```python
from build123d import *

# Parameters (mm, degrees)
SKETCH_1_W           = 36
SKETCH_1_H           = 219
EXTRUDE_1_DEPTH      = 37
SKETCH_2_W           = 80.767995678
SKETCH_2_H           = 159
CUT_EXTRUDE_1_DEPTH  = 117.975424769
CUT_EXTRUDE_START    = 10
SKETCH_9_W           = 26
SKETCH_9_H           = 219
CUT_EXTRUDE_7_DEPTH  = 17
SKETCH_10_W          = 12
SKETCH_10_H          = 236
CUT_EXTRUDE_8_DEPTH  = 17
CUT_EXTRUDE_START_2  = 37
SKETCH_11_R          = 3.5
CUT_EXTRUDE_11_DEPTH = 17
SKETCH_25_R          = 15
EXTRUDE_3_DEPTH      = 60
CUT_EXTRUDE_START_3  = -78
SKETCH_26_R          = 11
CUT_EXTRUDE_13_DEPTH = 3


with BuildPart() as part:
    # 스케치1 → 보스-돌출1 (new body)
    with BuildSketch(Plane.XY):
        Rectangle(SKETCH_1_W, SKETCH_1_H)
    extrude(amount=EXTRUDE_1_DEPTH)

    # 스케치2 → 컷-돌출1 (cut, through all)
    with BuildSketch(Plane.XY):
        with Locations((32.383997839, -3)):
            Rectangle(SKETCH_2_W, SKETCH_2_H)
    extrude(amount=CUT_EXTRUDE_1_DEPTH, mode=Mode.SUBTRACT)

    # 스케치9 → 컷-돌출7 (cut)
    with BuildSketch(Plane.XY.offset(CUT_EXTRUDE_START)):
        with Locations((5, 0)):
            Rectangle(SKETCH_9_W, SKETCH_9_H)
    extrude(amount=CUT_EXTRUDE_7_DEPTH, mode=Mode.SUBTRACT)

    # 스케치10 → 컷-돌출8 (cut)
    with BuildSketch(Plane.XY):
        with Locations((12, 8.5)):
            Rectangle(SKETCH_10_W, SKETCH_10_H)
    extrude(amount=CUT_EXTRUDE_8_DEPTH, mode=Mode.SUBTRACT)

    # 스케치11 → 컷-돌출11 (cut)
    with BuildSketch(Plane.XY.offset(CUT_EXTRUDE_START_2)):
        with Locations((3.878169626, 88)):
            Circle(SKETCH_11_R)
        with Locations((3.878169626, -92)):
            Circle(SKETCH_11_R)
    extrude(amount=-CUT_EXTRUDE_11_DEPTH, mode=Mode.SUBTRACT)

    # 스케치25 → 보스-돌출3 (add)
    with BuildSketch(Plane.ZY.offset(18)):
        with Locations(Location((18.5, 0, 0), (0, 0, 180))):
            Circle(SKETCH_25_R)
    extrude(amount=EXTRUDE_3_DEPTH)

    # 스케치26 → 컷-돌출13 (cut)
    with BuildSketch(Plane(origin=(0, 0, 0), x_dir=(0, 0, -1), z_dir=(1, 0, 0)).offset(CUT_EXTRUDE_START_3)):
        with Locations(Location((-18.5, 0, 0), (0, 0, 180))):
            Circle(SKETCH_26_R)
    extrude(amount=CUT_EXTRUDE_13_DEPTH, mode=Mode.SUBTRACT)


solid = part.part
```
The model under review builds one solid part; all positions refer to its coordinate system, in mm. A direction names the side the tool comes from. Give positions to 0.01 mm unless a question says otherwise; leave off trailing zeros. Write each loop counter-clockwise with the first axis right and the second up, starting at its lowest first coordinate (ties: lowest second). Pieces come first, ordered by that corner, then holes. Notation, with made-up numbers: (20.5, 19.25) - (62.5, 19.25) arc R26 cw to (62.5, 42.25) - close; hole circle Ø8 at (-1.5, -8.5). An arc over 180 degrees is marked (long way). Answer in a Markdown table with one row per item. Add a question column.
1. Insertion check: P1, Ø3, axis at y = -91, z = 5.5, coming from the +X side; P2, Ø2, axis at y = 10.5, z = 30, coming from the +X side; P3, Ø6, axis at x = -35.5, z = 22.5, coming from the -Y side. Each pin has a flat end and moves straight along its axis. Give the tip position at first contact, or say it passes through.
2. Wall thickness on line 1 along X through (y, z) = (-35, 3.5); line 2 along X through (y, z) = (-9, 17.5); line 3 along Y through (x, z) = (-47, 9): over which ranges is each line inside the solid? List them lowest first. Write a range as [from, to].
3. Tool access review of faces 1 (the flat face through (6, 93, 5)), 2 (the cylindrical face through (3.119, -95.417, 32.07)), 3 (the flat face through (-1, 76.5, 5)), 4 (the flat face through (-75, 0, 18)), 5 (the flat face through (-1, 93, 10)): name each direction out of +Z, -Z, +X, -X, +Y, -Y from which nothing blocks a thin tool from reaching the whole face with its end or side.
4. We need section D-D on y = 0. Write out the cut boundary in (x, z).
5. We need section B-B on y = -92. Write out the cut boundary in (x, z), then the cut area to 3 significant figures.
6. We need section A-A on x = 12. Write out the cut boundary in (y, z), then the cut area to 3 significant figures.
7. Draft analysis for pull direction Y (two halves, no side actions). For faces 6 (the flat face through (-8.3, 109.5, 18.2)), 7 (the cylindrical face through (-76.521, 4.213, 28.661)), 8 (the flat face through (5, -96, 27)), state which applies: +Y half, -Y half, draft (parallel to the pull), parting line (faces both ways), or undercut.
8. We need section C-C on z = 18.5. Write out the cut boundary in (x, y), then the cut area to 3 significant figures.
Ans:
| question | item | result |
|---|---|---|
| 1 | P1 | stops at x = 6 |
| 1 | P2 | stops at x = -8 |
| 1 | P3 | stops at y = -14.97 |
| 2 | line 1 | x = [-18, -8] |
| 2 | line 2 | x = [-75, -8] |
| 2 | line 3 | y = [-11.61, 11.61] |
| 3 | face 1 | -Z, +X, +Y, -Y |
| 3 | face 2 | +Z |
| 3 | face 3 | +Z, -Z, +X |
| 3 | face 4 | -X |
| 3 | face 5 | +X, +Y, -Y |
| 4 | outline | (-78, 3.5) - (-18, 3.5) - (-18, 0) - (-8, 0) - (-8, 37) - (-18, 37) - (-18, 33.5) - (-78, 33.5) - (-78, 29.5) - (-75, 29.5) - (-75, 7.5) - (-78, 7.5) - close |
| 5 | outline | (-18, 0) - (6, 0) - (6, 10) - (-8, 10) - (-8, 27) - (0.38, 27) - (0.38, 37) - (-18, 37) - close; (7.38, 27) - (18, 27) - (18, 37) - (7.38, 37) - close |
| 5 | area | 700 mm^2 |
| 6 | outline | (-109.5, 27) - (-82.5, 27) - (-82.5, 37) - (-109.5, 37) - close; (76.5, 27) - (109.5, 27) - (109.5, 37) - (76.5, 37) - close |
| 6 | area | 600 mm^2 |
| 7 | face 6 | +Y half |
| 7 | face 7 | undercut |
| 7 | face 8 | draft |
| 8 | outline | (-78, -15) - (-18, -15) - (-18, -109.5) - (-8, -109.5) - (-8, 109.5) - (-18, 109.5) - (-18, 15) - (-78, 15) - (-78, 11) - (-75, 11) - (-75, -11) - (-78, -11) - close |
| 8 | area | 3,920 mm^2 |
